Input: dimensioned drawing with shaded views. Units: mm. Origin: part minimum x, y, z. Coordinates: 2 decimals unless noted, no trailing zeros. Write each loop counter-clockwise with the first axis right and the second up, starting at its lowest first coordinate (ties: lowest second). Pieces come first, ordered by that corner, then holes. Notation, with made-up numbers: (85, 78.25) - (129, 78.25) arc R19 cw to (129, 93.25) - close; hole circle Ø11 at (47.25, 39.5). An arc over 180 degrees is marked (long way). One line per question, with ' | ' between items.
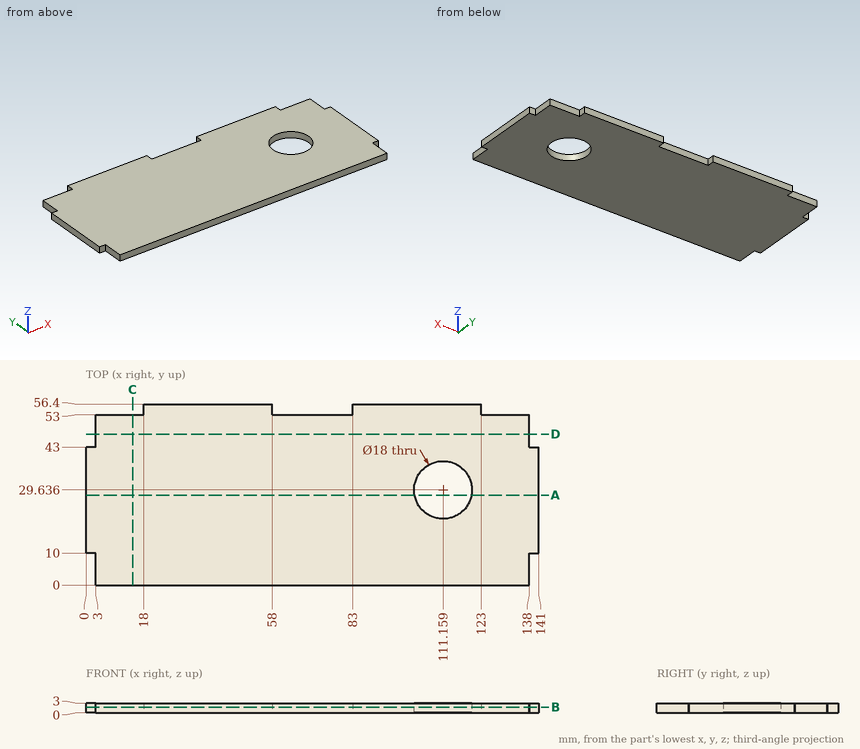
Item 1: Pin query (flat end, axial travel): pin 1 Ø0.9 at (x, z) = (129.5, 2) entering from +Y; pin 2 Ø0.9 at (y, z) = (55, 2) entering from +X; pin 3 Ø1.5 at (x, z) = (2, 1) entering from -Y; pin 4 Ø10 at (x, y) = (63.5, 11) entering from -Z. Return the tip coordinate at first contact, or that it passes through.
Check sheet entries:
pin 1: y = 53 | pin 2: x = 123 | pin 3: y = 10 | pin 4: z = 0
Item 2: Cut plane C-C on x = 14.5. Return loops of the section in (y, z).
Check sheet entries:
outline: (0, 0) - (53, 0) - (53, 3) - (0, 3) - close
Item 3: Cut plane D-D on y = 47. Return loops of the section in (x, z), and give its area (3 significant figures).
Check sheet entries:
outline: (3, 0) - (138, 0) - (138, 3) - (3, 3) - close | area: 405 mm²
Item 4: Ray query, line 1 along X through (y, z) = (30, 2); line 2 along X through (y, z) = (7, 0.45); line 3 along Y through (x, z) = (15.5, 1.05). Return the intervals inside material, ascending. Write a range as [from, to].
Check sheet entries:
line 1: [0, 102.17], [120.15, 141] | line 2: [3, 138] | line 3: [0, 53]
Item 5: Cut plane A-A on y = 28. Return loops of the section in (x, z), and give its area (3 significant figures).
Check sheet entries:
outline: (0, 0) - (102.31, 0) - (102.31, 3) - (0, 3) - close; (120.01, 0) - (141, 0) - (141, 3) - (120.01, 3) - close | area: 370 mm²
Item 6: Cut plane B-B on z = 1.75. Return loops of the section in (x, y), and give its area (3 significant figures).
Check sheet entries:
outline: (0, 10) - (3, 10) - (3, 0) - (138, 0) - (138, 10) - (141, 10) - (141, 43) - (138, 43) - (138, 53) - (123, 53) - (123, 56.4) - (83, 56.4) - (83, 53) - (58, 53) - (58, 56.4) - (18, 56.4) - (18, 53) - (3, 53) - (3, 43) - (0, 43) - close; hole circle Ø18 at (111.16, 29.64) | area: 7,370 mm²
